Part model, mm, in its own coordinate system. Give positions to 0.01 mm unless a question says otherwise; leave off trailing zeros. Order: outer loops, then holes, each group sorted by start corner. A loop starts at its lowest first (then second) coordinate and runs counter-clockwise, first axis right, second up. Notation, with made-up numbers: M 66,-31 L 118,-31 A21 ccw 118,-18 Z; hole C 57,63 d11. An arc over 180 degrees is marked long. Answer as a JSON object with one key per item and string values.
from build123d import *

# Parameters (mm, degrees)
F0_W     = 50
F0_H     = 50
F0_W_2   = 46.8
F0_H_2   = 46.8
F1_DEPTH = 757
F2_W     = 50
F2_H     = 50
F2_W_2   = 46.8
F2_H_2   = 46.8
F3_DEPTH = 325
F4_W     = 75
F4_H     = 50
F5_DEPTH = 3
F6_W     = 50
F6_H     = 50
F6_W_2   = 46.8
F6_H_2   = 46.8
F7_DEPTH = 922
F9_DEPTH = 922


with BuildPart() as f1:
    # F0 (on Top) → F1 (new body)
    with BuildSketch(Plane.XY):
        with Locations((-25, 41.517847)):
            Rectangle(F0_W, F0_H)
        with Locations((-25, 41.517847)):
            Rectangle(F0_W_2, F0_H_2, mode=Mode.SUBTRACT)
    extrude(amount=F1_DEPTH)

    # F2 (on face) → F3 (join)
    with BuildSketch(Plane.YZ):
        with Locations((41.517847, 732)):
            Rectangle(F2_W, F2_H)
        with Locations((41.517847, 732)):
            Rectangle(F2_W_2, F2_H_2, mode=Mode.SUBTRACT)
        with Locations((41.517847, 30)):
            Rectangle(F2_W, F2_H)
        with Locations((41.517847, 30)):
            Rectangle(F2_W_2, F2_H_2, mode=Mode.SUBTRACT)
    extrude(amount=F3_DEPTH)

    # F4 (on face) → F5 (join)
    with BuildSketch(Plane.XZ.offset(-16.517847)):
        Polygon((50, 757), (-50, 757), (-50, 657), (0, 657), (0, 707), (50, 707), align=None)
        with Locations((287.5, 30)):
            Rectangle(F4_W, F4_H)
    extrude(amount=F5_DEPTH)

    # F6 (on face) → F7 (join)
    with BuildSketch(Plane.XZ.offset(-13.517847)):
        with Locations((-25, 732)):
            Rectangle(F6_W, F6_H)
        with Locations((-25, 732)):
            Rectangle(F6_W_2, F6_H_2, mode=Mode.SUBTRACT)
    extrude(amount=F7_DEPTH)

    # F8 (on face) → F9 (join)
    with BuildSketch(Plane.XZ.offset(-13.517847)):
        Polygon((325, 53.4), (325, 55), (300, 55), (300, 5), (325, 5), (325, 6.6), (301.6, 6.6), (301.6, 53.4), align=None)
    extrude(amount=F9_DEPTH)

    # F10: F1 across face


with BuildPart() as f1_1:
    add(f1.part)
    add(f1.part.mirror(Plane(origin=(325, -382.720488, 30), x_dir=(0, 1, 0), z_dir=(1, 0, 0))))

    # F11: F1 across face


with BuildPart() as f1_2:
    add(f1_1.part)
    add(f1_1.part.mirror(Plane(origin=(325, -908.482153, 30), x_dir=(1, 0, 0), z_dir=(0, -1, 0))))


solid = f1_2.part
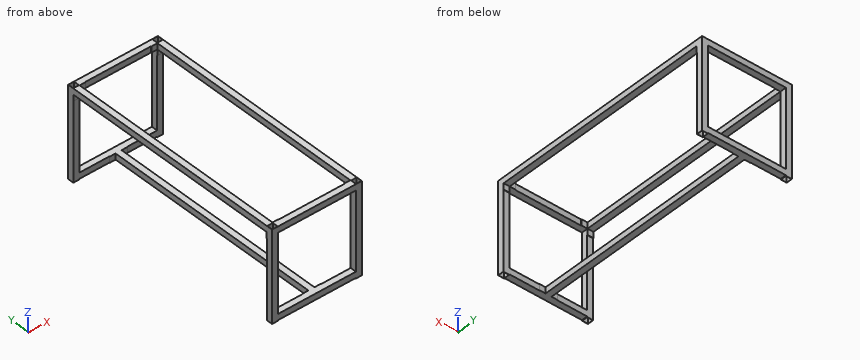
1. Cut at A-A on y = -167.5. Give the cut face in (x, z), plus the area to 3 significant figures.
Worked answers:
{"outline": "M -50,707 L 0,707 L 0,757 L -50,757 Z; M 300,5 L 350,5 L 350,55 L 300,55 Z; M 650,707 L 700,707 L 700,757 L 650,757 Z; hole M -48.4,708.6 L -1.6,708.6 L -1.6,755.4 L -48.4,755.4 Z; hole M 301.6,6.6 L 348.4,6.6 L 348.4,53.4 L 301.6,53.4 Z; hole M 651.6,708.6 L 698.4,708.6 L 698.4,755.4 L 651.6,755.4 Z", "area": "929 mm^2"}
2. Pin check, flat tips, straight feed: P1, Ø23.5, axis at y = -1132, z = 27, coming from the -X side; P2, Ø14, axis at x = 292, y = -1861, coming from the -Z side. Stop position of each tip, or through.
Worked answers:
{"P1": "stops at x = 300", "P2": "stops at z = 5"}
3. Cut at B-B on z = 419. State how many separate pieces and enclosed holes the cut face has, plus the area to 3 significant figures.
Worked answers:
{"separate pieces": "4", "enclosed holes": "4", "area": "1,240 mm^2"}
4. Probe line 1 along Y through (x, z) = (667.5, 309); line 2 along Z through (x, y) = (339.5, -1468.5); line 3 along Z through (x, y) = (661.5, -778). List the from-to ranges inside material, lowest first.
Worked answers:
{"line 1": "y = -1883.48 to -1881.88, -1835.08 to -1833.48, 16.52 to 18.12, 64.92 to 66.52", "line 2": "z = 5 to 6.6, 53.4 to 55", "line 3": "z = 707 to 708.6, 755.4 to 757"}
